CAD build for the part. Positions are in the model's coordinates, mm. Face numbers are marked on the shaded views. Give positions to 0.01 mm unless a question says otherwise; leave off trailing zeros. Loops run counter-clockwise (first coordinate to the right, second up) from the corner with the lowest first, then second, coordinate; pieces in that order, holes last. Notation, with made-up numbers: (-23.5, 36.5) - (26.5, 36.5) arc R18 ccw to (26.5, 52.5) - close; hole circle Ø7 at (-14.5, -26). An arc over 180 degrees is marked (long way). Return JSON: item names as keys, results as strings.
Autodesk Inventor part; units mm, degrees
ref_plane "YZ Plane" through (0, 0, 0) normal (1, 0, 0) x (0, 1, 0)
ref_plane "XZ Plane" through (0, 0, 0) normal (0, 1, 0) x (-1, 0, 0)
ref_plane "XY Plane" through (0, 0, 0) normal (0, 0, 1) x (1, 0, 0)
sketch "スケッチ1" plane through (0, 0, 0) normal (0, 0, 1) x (1, 0, 0)
  line L0 (-170.6512, -31.4118) -> (202.8656, -31.4118) construction
  circle A0 centre (-14, -17.4118) radius 14 construction
  circle A1 centre (14, -17.4118) radius 14 construction
  circle A2 centre (-28.0204, 0.0121) radius 20.05 construction
  circle A3 centre (-28.0204, 0.0121) radius 5.05 construction
  circle A4 centre (8.8763, 3.8907) radius 32.05 construction
  circle A5 centre (8.8763, 3.8907) radius 10.1 construction
  circle A6 centre (54.047, 13.5882) radius 36.1 construction
  line L1 (-170.915, -81.4118) -> (490.0044, -81.4118)
  circle A7 centre (-28.0204, 0.0121) radius 22.342 construction
  circle A8 centre (-39.4931, 19.1835) radius 14 construction
  circle A9 centre (-49.0547, 7.5438) radius 14 construction
  circle A10 centre (-49.0547, -7.5196) radius 14 construction
  circle A11 centre (-39.4931, -19.1593) radius 14 construction
  circle A12 centre (8.8763, 3.8907) radius 33.05 construction
  circle A13 centre (54.047, 13.5882) radius 38.1 construction
  line L2 (-11.5565, -29.1593) -> (4.2969, -29.1593) construction
  line L3 (-67.2952, 44.8622) -> (-67.2952, -57.3934) construction
  line L4 (-149.4523, -1.6098) -> (-132.6633, -31.6026)
  line L5 (-132.7701, -31.4118) -> (-132.7701, 74.0456)
  circle A14 centre (-11.4931, -19.1593) radius 14 construction
  line L6 (-197.2268, -33.1593) -> (179.6604, -33.1593) construction
  circle A15 centre (54.047, 13.5882) radius 4.025
  circle A16 centre (54.047, 13.5882) radius 6
  circle A17 centre (-39.4931, 19.1835) radius 5
  circle A18 centre (-49.0547, 7.5438) radius 5
  circle A19 centre (-49.0547, -7.5196) radius 5
  circle A20 centre (-39.4931, -19.1593) radius 5
  circle A21 centre (-39.4931, 19.1835) radius 8 construction
  circle A22 centre (-49.0547, 7.5438) radius 8 construction
  circle A23 centre (-49.0547, -7.5196) radius 8 construction
  circle A24 centre (-39.4931, -19.1593) radius 8 construction
  circle A25 centre (-28.0204, 0.0121) radius 4.5
  circle A26 centre (8.8763, 3.8907) radius 7.5
  line L7 (-17.5497, 32.3149) -> (-46.3578, 15.0755) construction
  line L8 (-46.3578, 15.0755) -> (-51.7515, 0.0121) construction
  line L9 (-51.7515, 0.0121) -> (-46.3578, -15.0513) construction
  line L10 (-46.3578, -15.0513) -> (-37.9391, -20.0892) construction
  circle A27 centre (-32.6283, 23.2915) radius 1.3
  circle A28 centre (-46.3578, 15.0755) radius 1.3
  circle A29 centre (-51.7515, 0.0121) radius 1.3
  circle A30 centre (-46.3578, -15.0513) radius 1.3
  circle A31 centre (-32.6283, -23.2673) radius 1.3
  line L11 (-67.2952, 23.1796) -> (-67.2952, -18.1327)
  arc A32 (79.2003, -37.212) -> (87.3507, -31.2711) centre (80.4159, -30.3183) ccw
  arc A33 (8.1864, 50.8943) -> (0.9804, 51.9708) centre (3.7003, 45.5208) ccw
  line L12 (-52.2685, -33.1593) -> (56.2168, -33.1593)
  line L13 (56.2168, -33.1593) -> (79.2003, -37.212)
  arc A34 (92.7831, 8.2659) -> (29.742, 44.2162) centre (54.047, 13.5882) ccw
  line L14 (87.3507, -31.2711) -> (92.7831, 8.2659)
  line L15 (0.9804, 51.9708) -> (-67.2952, 23.1796)
  circle A35 centre (34.0114, -24.0061) radius 4.5 construction
  circle A36 centre (34.0114, -24.0061) radius 1.5
  circle A37 centre (-21.4477, 26.0369) radius 4.5 construction
  circle A38 centre (-21.4477, 26.0369) radius 1.5
  circle A39 centre (-56.0504, 23.0377) radius 1.5
  circle A40 centre (-56.0504, 23.0377) radius 3 construction
  circle A41 centre (-56.0504, 23.0377) radius 4.5 construction
  circle A42 centre (-64.2952, 0.0121) radius 1.5
  circle A43 centre (-64.2952, 0.0121) radius 3 construction
  circle A44 centre (-64.2952, 0.0121) radius 4.3311 construction
  line L16 (54.047, 13.5882) -> (99.37, -7.5264)
  line L17 (99.37, -7.5264) -> (58.3399, 10.9541)
  line L18 (58.3399, 10.9541) -> (30.7326, 32.4678)
  line L19 (30.7326, 32.4678) -> (54.047, 13.5882)
  line L20 (99.37, -7.5264) -> (491.4359, -184.1173)
  line L21 (-183.2789, 162.2213) -> (-183.2789, -125.2315)
  line L22 (516.7211, 155.5913) -> (516.7211, -155.5644)
  circle A45 centre (99.37, -7.5264) radius 7.25
  line L23 (135.8413, -23.9534) -> (383.826, -192.7834) construction
  line L24 (218.8627, -80.4751) -> (224.047, -10.6673) construction
  circle A46 centre (3.7003, 45.5208) radius 4
  circle A47 centre (122.1646, -17.7933) radius 2
  circle A48 centre (135.8413, -23.9534) radius 2
  arc A49 (134.404, -28.7424) -> (138.4753, -19.7035) centre (135.8413, -23.9534) ccw
  line L25 (134.404, -28.7424) -> (96.4236, -17.3438)
  line L26 (138.4753, -19.7035) -> (104.7697, 1.1861)
  circle A50 centre (30.7326, 32.4678) radius 2
  circle A51 centre (-16.1798, -24.0771) radius 4.5 construction
  circle A52 centre (-16.1798, -24.0771) radius 1.5
  line L27 (-67.2952, -18.1327) -> (-52.2685, -33.1593)
  circle A53 centre (-56.0504, -23.0135) radius 1.5
  circle A54 centre (-56.0504, -23.0135) radius 3 construction
  circle A55 centre (30.7326, 32.4678) radius 4
  arc A56 (56.8403, 15.6972) -> (51.3644, 11.3402) centre (54.047, 13.5882) ccw
  line L28 (96.4916, -6.1854) -> (101.9705, -5.7041) construction
  line L29 (101.9705, -5.7041) -> (99.6479, -10.6896) construction
  line L30 (99.6479, -10.6896) -> (96.4916, -6.1854) construction
  circle A57 centre (99.6479, -10.6896) radius 1.5
  circle A58 centre (101.9705, -5.7041) radius 1.5
  circle A59 centre (96.4916, -6.1854) radius 1.5
  circle A60 centre (99.37, -7.5264) radius 6
  arc A61 (97.7876, -15.8778) -> (97.5111, 0.7679) centre (99.37, -7.5264) ccw
  arc A62 (56.8403, 15.6972) -> (97.5111, 0.7679) centre (88.7632, 39.7996) ccw
  arc A63 (51.3644, 11.3402) -> (97.7876, -15.8778) centre (112.6811, 62.7237) ccw
  circle A64 centre (54.047, 13.5882) radius 8.5
  line L31 (102.9595, 0.1786) -> (57.6365, 21.2931)
  line L32 (50.4575, 5.8833) -> (95.7806, -15.2313)
  circle A65 centre (12.7384, 41.2415) radius 3 construction
  circle A66 centre (12.7384, 41.2415) radius 4.5 construction
  circle A67 centre (12.7384, 41.2415) radius 1.5
  circle A68 centre (80.4159, -30.3183) radius 4
  circle A69 centre (69.7531, -26.0108) radius 1.5
  circle A70 centre (69.7531, -26.0108) radius 4.5 construction
  circle A71 centre (-56.0504, -23.0135) radius 4.5 construction
  line L33 (8.1864, 50.8943) -> (15.9809, 44.3871)
  arc A72 (15.9809, 44.3871) -> (29.742, 44.2162) centre (22.9664, 52.7545) ccw
  circle A73 centre (-5.4761, 38.5895) radius 1.5
  circle A74 centre (-5.4761, 38.5895) radius 4.5 construction
  circle A75 centre (54.047, 13.5882) radius 50 construction
  circle A76 centre (3.7003, 45.5208) radius 2
  circle A77 centre (80.4159, -30.3183) radius 2
  circle A78 centre (54.047, 13.5882) radius 1.5 construction
  circle A79 centre (58.3399, 10.9541) radius 1.5
  circle A80 centre (58.3399, 10.9541) radius 3
  circle A81 centre (58.3399, 10.9541) radius 5
  line L34 (94.099, -16.3172) -> (55.7687, 6.6659)
  line L35 (59.8474, 15.7214) -> (102.4604, 2.2467)
  arc A82 (104.7697, 1.1861) -> (102.4604, 2.2467) centre (99.37, -7.5264) ccw
  arc A83 (94.099, -16.3172) -> (96.4236, -17.3438) centre (99.37, -7.5264) ccw
  circle A84 centre (30.7326, 32.4678) radius 5.025
  circle A85 centre (30.7326, 32.4678) radius 8.025
  circle A86 centre (58.3399, 10.9541) radius 4.025
  circle A87 centre (58.3399, 10.9541) radius 7.025
  line L36 (25.9827, 25.9995) -> (54.1819, 5.2918)
  line L37 (53.3095, 15.8577) -> (37.1861, 27.6978)
  line L38 (65.3516, 11.3852) -> (66.2721, -3.5865)
  line L39 (66.2721, -3.5865) -> (54.1819, 5.2918)
  point P0 (0, 0)
  point P1 (0, 0)
  point P2 (-49.0547, 7.5438)
  point P3 (-49.0547, -7.5196)
  dimension "d88" = 100
  dimension "d0" = 40.1
  dimension "d1" = 10.1
  dimension "d2" = 64.1
  dimension "d3" = 20.2
  dimension "d4" = 72.2
  dimension "d5" = 95
  dimension "d6" = 44.684
  dimension "d7" = 28
  dimension "d8" = 28
  dimension "d9" = 28
  dimension "d10" = 28
  dimension "d11" = 1
  dimension "d12" = 2
  dimension "d13" = 4
  dimension "d14" = 8.05
  dimension "d15" = 12
  dimension "d16" = 10
  dimension "d17" = 10
  dimension "d18" = 10
  dimension "d19" = 10
  dimension "d20" = 3
  dimension "d21" = 3
  dimension "d22" = 3
  dimension "d23" = 3
  dimension "d24" = 9
  dimension "d25" = 15
  dimension "d26" = 2.6
  dimension "d27" = 2.6
  dimension "d28" = 2.6
  dimension "d29" = 2.6
  dimension "d30" = 2.6
  dimension "d31" = 1
  dimension "d32" = 9
  dimension "d33" = 3
  dimension "d34" = 9
  dimension "d35" = 3
  dimension "d36" = 3
  dimension "d37" = 6
  dimension "d38" = 9
  dimension "d39" = 3
  dimension "d40" = 6
  dimension "d41" = 50
  dimension "d42" = 45
  dimension "d43" = 35
  dimension "d44" = 30
  dimension "d45" = 39
  dimension "d46" = 430
  dimension "d47" = 700
  dimension "d48" = 14.5
  dimension "d49" = 300
  dimension "d50" = 10
  dimension "d51" = 70
  dimension "d52" = 120
  dimension "d53" = 140
  dimension "d54" = 8
  dimension "d55" = 4
  dimension "d56" = 4
  dimension "d57" = 15
  dimension "d58" = 25
  dimension "d59" = 10
  dimension "d60" = 4
  dimension "d61" = 9
  dimension "d62" = 3
  dimension "d63" = 3
extrude "押し出し1" add sketch "スケッチ1" along normal blind 3 contours A86 A62 A56 A81 A15 | A15 A81 A16 A86 | A86 L18 A81 A56 A62 | A86 L16 A81 L18 | A81 A56 A87 A15 | A15 A87 A16 A81 | A16 A81 A64 A86 | A81 L16 L19 A87 L18 | L18 A87 A56 A81 | A86 A15 A81 L16 | A16 A87 A64 L35 A81 | A64 A81 L16 A62 A86 | A87 L19 A56 L18 | L18 A56 L37 A87 | A81 A15 A63 A56 A87 L19 L16 | A86 A16 A63 A81 A15 | L37 A56 L18 A15 | A15 L18 A16 L37 | L35 A64 A81 | A62 L16 A86 | A56 L19 A15 L18 | A87 A56 L19 | A81 A63 A15 | A86 A64 A81 A63 A16 | A15 L19 A16 L18 | A16 L18 A64 L37 | A87 L35 A64 | A64 L35 A87 L16 A81 | A62 A81 L17 A86 L16 | L16 A81 A62 | A56 A87 A15 L19 | A56 A63 A15 A87 | A63 A81 A16 A87 A15 | A63 A16 A81 | A63 A81 A16 | A86 L17 A81 A64 | A15 A87 A16 L19 | A16 L19 A64 L18 | A64 L18 A85 L37 | L16 A87 L17 A62 A81 | A62 L17 A81 | A81 A63 A64 A87 A16 | A81 L34 A64 A63 | A81 L17 A62 A87 L34 A64 | A64 L34 A81 | A16 A87 L36 A64 L19 | A64 L19 A85 L18 | A85 L18 A84 L19 | L38 L16 A87 | L16 L38 L17 A87 | L17 A87 A62 | A64 L34 A87 A63 | A63 A87 A64 | A64 L36 A85 L19 | A85 L19 A84 L18 | L17 L38 A62 A87 | A62 L38 L34 A87 | A87 A64 L39 | A87 L34 L38 L32 A63 | A63 L32 L39 A64 A87 | L32 L38 A63 | A63 L38 L39 L32
fillet "フィレット1" radius 5 2 edges at (37.1861, 27.6978, 1.5) (53.3095, 15.8577, 1.5)
properties part number "アーム揺動節" material "アルミニウム 7075"
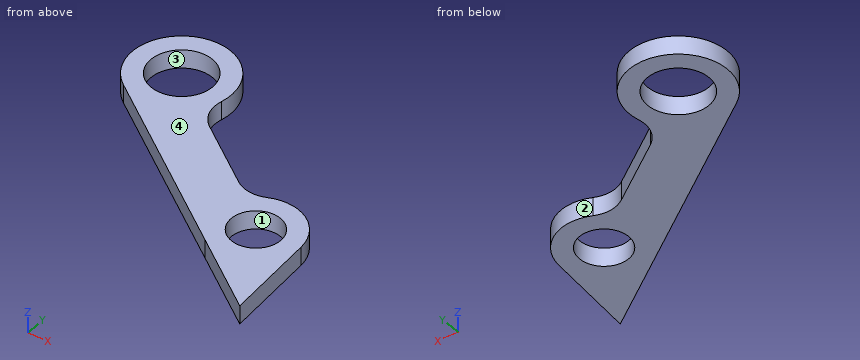
1. Cut at D-D, the plane y = 1. Write the cut outline in (x, z).
Values follow:
{"outline": "(60.03, 0) - (65.99, 0) - (65.99, 3) - (60.03, 3) - close"}
2. Cut at B-B, the plane y = 8.5. Write the cut outline in (x, z).
Values follow:
{"outline": "(49.81, 0) - (55.15, 0) - (55.15, 3) - (49.81, 3) - close; (61.53, 0) - (65.53, 0) - (65.53, 3) - (61.53, 3) - close"}
3. Drill centre lines: probe 1 along X at (y, z) = (33, 1.75); probe 2 along X at (y, z) = (14, 2.75); probe 3 along Y at (x, z) = (61.5, 2.35). Where is each one in solid material? Low to high.
Values follow:
{"probe 1": "x = 22.73 to 25.74, 35.73 to 38.74", "probe 2": "x = 42.32 to 55.71, 60.97 to 64.67", "probe 3": "y = -0.08 to 8.46, 13.45 to 17.23"}
4. Cut at A-A, the plane x = 34. Write the cut outline in (y, z).
Values follow:
{"outline": "(20.11, 0) - (28.65, 0) - (28.65, 3) - (20.11, 3) - close; (36.29, 0) - (39.8, 0) - (39.8, 3) - (36.29, 3) - close"}
5. Pull direction Y, two halves, no side cores. Call the marked faces 1, 2, 3 and 4: +Y half, -Y half, draft (parallel to the pull), parting line (faces both ways), or undercut.
Values follow:
{"face 1": "undercut", "face 2": "+Y half", "face 3": "undercut", "face 4": "draft"}
6. Cut at C-C, the plane z = 2.1. Give the number of separate pieces and of enclosed holes in the cut face, plus the area to 3 significant figures.
Values follow:
{"separate pieces": "1", "enclosed holes": "2", "area": "465 mm²"}
